Here's how the part is built. I have some questions about the finished solid (model axes, mm). A direction names the side the tool comes from. Coordinates: 2 decimals unless noted, no trailing zeros. Write each loop counter-clockwise with the first axis right and the second up, starting at its lowest first coordinate (ties: lowest second). Pieces come first, ordered by that corner, then holes.
from build123d import *

# Parameters (mm, degrees)
CROQUIS1_W              = 30
CROQUIS1_H              = 10
SALIENTE_EXTRUIR1_DEPTH = 30
CORTAR_EXTRUIR1_REACH   = 45.589
CROQUIS2_W              = 20
CROQUIS2_H              = 7
CROQUIS4_W              = 26
CROQUIS4_H              = 24
CORTAR_EXTRUIR3_DEPTH   = 7
CORTAR_EXTRUIR4_REACH   = 43.581
CROQUIS5_R              = 2.5
CROQUIS6_W              = 30
CROQUIS6_H              = 10
CORTAR_EXTRUIR5_DEPTH   = 3


with BuildPart() as part:
    # Croquis1 → Saliente-Extruir1 (new body)
    with BuildSketch(Plane(origin=(0, 0, 0), x_dir=(1, 0, 0), z_dir=(0, 1, 0))):
        with Locations((-15, -5)):
            Rectangle(CROQUIS1_W, CROQUIS1_H)
    extrude(amount=SALIENTE_EXTRUIR1_DEPTH)

    # Croquis2 → Cortar-Extruir1 (cut, up to next)
    with BuildSketch(Plane.XY.offset(10), mode=Mode.PRIVATE) as cortar_extruir1_sk1:
        with Locations((-15, 16)):
            Rectangle(CROQUIS2_W, CROQUIS2_H)
    cortar_extruir1_tool1 = extrude(cortar_extruir1_sk1.sketch, amount=-CORTAR_EXTRUIR1_REACH, mode=Mode.PRIVATE) & part.part
    add(cortar_extruir1_tool1.solids().sort_by_distance((-15, 16, 10))[0], mode=Mode.SUBTRACT)

    # Croquis4 → Cortar-Extruir3 (cut)
    with BuildSketch(Plane(origin=(0, 0, 0), x_dir=(-1, 0, 0), z_dir=(0, 0, -1))):
        with Locations((15, 15)):
            Rectangle(CROQUIS4_W, CROQUIS4_H)
    extrude(amount=-CORTAR_EXTRUIR3_DEPTH, mode=Mode.SUBTRACT)

    # Croquis5 → Cortar-Extruir4 (cut, up to next)
    with BuildSketch(Plane(origin=(0, 3, 0), x_dir=(1, 0, 0), z_dir=(0, 1, 0)), mode=Mode.PRIVATE) as cortar_extruir4_sk1:
        with Locations((-15, 0)):
            Circle(CROQUIS5_R)
    cortar_extruir4_tool1 = extrude(cortar_extruir4_sk1.sketch, amount=-CORTAR_EXTRUIR4_REACH, mode=Mode.PRIVATE) & part.part
    add(cortar_extruir4_tool1.solids().sort_by_distance((-15, 3, 0))[0], mode=Mode.SUBTRACT)

    # Croquis6 → Cortar-Extruir5 (cut)
    with BuildSketch(Plane(origin=(0, 30, 0), x_dir=(1, 0, 0), z_dir=(0, 1, 0))):
        with Locations((-15, -5)):
            Rectangle(CROQUIS6_W, CROQUIS6_H)
    extrude(amount=-CORTAR_EXTRUIR5_DEPTH, mode=Mode.SUBTRACT)


solid = part.part
1. Thinking about a two-plate mould opening in X: for faces 1 (the face through (0, 13, 5)), 2 (the face through (-30, 13, 5)), 3 (the face through (-15.2, 27, 7.2)), 4 (the face through (-5, 16, 9)), which applies, pulls with the +X half, pulls with the -X half, needs draft (parallel to the pull), parting line crosses it, or undercut?
2. I want a section at C-C (z = 2). List the corners of the cut face in (x, y) for me.
3. For pin 1 Ø7 at (x, y) = (-18.5, 18.5) entering from -Z, with a flat end and sliding along its axis, tell me the tip position at first contact or that it passes through.
4. On a 3-axis mill with a long thin cutter (end or side, diameter ignored), from which of +Z, -Z, +X, -X, +Y, -Y can I reach the whole of each face in a straight line? I mean faces 5 (the face through (-15, 3, 3)), 6 (the face through (-1.6, 8.4, 0)), 7 (the face through (-15, 12.5, 9)). Say none if no direction works.
5. I want a section at A-A (x = -12). List the corners of the cut face in (y, z) for me.
6. If I drill on line 1 (X direction, y = 18.5, z = 8.5); line 2 (X direction, y = 10, z = 5); line 3 (Y direction, x = -7.5, z = 8.25), over which ranges is the centre line in solid material (lowest first)?
7. I want a section at D-D (x = -15). List the corners of the cut face in (y, z) for me.
8. I want a section at B-B (y = 16.25). List the corners of the cut face in (x, z) for me, then the cut area to 3 significant figures.
Response values:
1. face 1: pulls with the +X half
1. face 2: pulls with the -X half
1. face 3: needs draft
1. face 4: undercut
2. outline: (-30, 0) - (-16.5, 0) - (-16.5, 3) - (-28, 3) - (-28, 27) - (-30, 27) - close; (-13.5, 0) - (0, 0) - (0, 27) - (-2, 27) - (-2, 3) - (-13.5, 3) - close
3. pin 1: stops at z = 7
4. face 5: -Z, +Y
4. face 6: -Z, +X, -X, +Y, -Y
4. face 7: +Z, -Z
5. outline: (0, 0) - (3, 0) - (3, 7) - (12.5, 7) - (12.5, 10) - (0, 10) - close; (19.5, 7) - (27, 7) - (27, 10) - (19.5, 10) - close
6. line 1: x = -30 to -25, -5 to 0
6. line 2: x = -30 to -28, -2 to 0
6. line 3: y = 0 to 12.5, 19.5 to 27
7. outline: (0, 2.5) - (3, 2.5) - (3, 7) - (12.5, 7) - (12.5, 10) - (0, 10) - close; (19.5, 7) - (27, 7) - (27, 10) - (19.5, 10) - close
8. outline: (-30, 0) - (-28, 0) - (-28, 7) - (-25, 7) - (-25, 10) - (-30, 10) - close; (-5, 7) - (-2, 7) - (-2, 0) - (0, 0) - (0, 10) - (-5, 10) - close
8. area: 58.0 mm2
